from build123d import *

# Parameters (mm, degrees)
SKETCH1_W                = 38
SKETCH1_H                = 20
BOSS_EXTRUDE1_DEPTH      = 3
M3_CLEARANCE_HOLE1_D     = 3.2
M3_CLEARANCE_HOLE1_DEPTH = 20
M3_CLEARANCE_HOLE1_TIP   = 0.96137699
CUT_EXTRUDE1_DEPTH       = 3
FILLET1_R                = 1


with BuildPart() as part:
    # Sketch1 → Boss-Extrude1 (new body)
    with BuildSketch(Plane.XY):
        with Locations((-19, 10)):
            Rectangle(SKETCH1_W, SKETCH1_H)
    extrude(amount=BOSS_EXTRUDE1_DEPTH)

    # M3 Clearance Hole1
    with Locations(Plane.XY.offset(3)):
        with Locations((-11.25, 16), (-26.75, 16)):
            Hole(M3_CLEARANCE_HOLE1_D / 2, depth=M3_CLEARANCE_HOLE1_DEPTH)
            with Locations((0, 0, -(M3_CLEARANCE_HOLE1_DEPTH + M3_CLEARANCE_HOLE1_TIP / 2))):  # 118° drill point
                Cone(0, M3_CLEARANCE_HOLE1_D / 2, M3_CLEARANCE_HOLE1_TIP, mode=Mode.SUBTRACT)

    # Sketch4 → Cut-Extrude1 (cut)
    with BuildSketch(Plane.XY.offset(3)):
        with BuildLine():
            Line((-9.75, 5.03), (-28.25, 5.03))
            ThreePointArc((-28.25, 5.03), (-29.25, 4.03), (-28.25, 3.03))
            Line((-28.25, 3.03), (-9.75, 3.03))
            ThreePointArc((-9.75, 3.03), (-8.75, 4.03), (-9.75, 5.03))
        make_face()
    extrude(amount=-CUT_EXTRUDE1_DEPTH, mode=Mode.SUBTRACT)

    # Fillet1
    fillet1_edges = [part.edges().sort_by_distance(p)[0] for p in [
        (0, 0, 1.5),
        (-38, 0, 1.5),
        (-38, 20, 1.5),
        (0, 20, 1.5),
    ]]
    fillet(fillet1_edges, radius=FILLET1_R)


solid = part.part
Geometry: final body of the model. Coordinates: model frame, mm. A direction names the side the tool comes from. Round coordinates to 2 decimals unless told otherwise and drop trailing zeros. Loops run counter-clockwise (first coordinate to the right, second up) from the corner with the lowest first, then second, coordinate; pieces in that order, holes last.
Q1. Section D-D on y = 16. Return loops of the section in (x, z).
Q2. Section C-C on z = 1.2. Return loops of the section in (x, y).
Q3. Pull-direction query (X, two-part tool) for faces 3 (the cylindrical face through (-0.301, 0.285, 1.521)), 4 (the cylindrical face through (-37.715, 19.699, 1.521)), 5 (the flat face through (-19, 3.03, 2)); classes: released by +X, released by -X, zero draft, split by the parting line, or undercut.
Q4. Section A-A on x = -21. Return loops of the section in (y, z).
Q5. Section B-B on y = 4.03. Return loops of the section in (x, z).
Q6. Material intervals for L1, parallel to Y at x = -26.75, z = 1.8; L2, parallel to Y at x = -21, z = 0.3; L3, parallel to X at y = 4.75, z = 0.6, sorted ascending.
Q7. Access query for faces 1 (the flat face through (-19, 20, 1)), 2 (the cylindrical face through (-8.75, 4.01, 1.52)). Directions: +Z, -Z, +X, -X, +Y, -Y. A direction counts if a zero-diameter tool reaches every point of the face in a straight line with its end or side. Return the directions, or none.
Q8. Pin query (flat end, axial travel): P1, Ø12, axis at x = -21, y = 7, coming from the -Z side; P2, Ø3, axis at x = -11.25, y = 16, coming from the +Z side. Return the tip coordinate at first contact, or that it passes through.
Evaluation:
1. outline: (-38, 0) - (-28.35, 0) - (-28.35, 3) - (-38, 3) - close; (-25.15, 0) - (-12.85, 0) - (-12.85, 3) - (-25.15, 3) - close; (-9.65, 0) - (0, 0) - (0, 3) - (-9.65, 3) - close
2. outline: (-38, 1) arc R1 ccw to (-37, 0) - (-1, 0) arc R1 ccw to (0, 1) - (0, 19) arc R1 ccw to (-1, 20) - (-37, 20) arc R1 ccw to (-38, 19) - close; hole circle Ø3.2 at (-26.75, 16); hole (-28.25, 3.03) - (-9.75, 3.03) arc R1 ccw to (-9.75, 5.03) - (-28.25, 5.03) arc R1 ccw to start; hole circle Ø3.2 at (-11.25, 16)
3. face 3: released by +X
3. face 4: released by -X
3. face 5: undercut
4. outline: (0, 0) - (3.03, 0) - (3.03, 3) - (0, 3) - close; (5.03, 0) - (20, 0) - (20, 3) - (5.03, 3) - close
5. outline: (-38, 0) - (-29.25, 0) - (-29.25, 3) - (-38, 3) - close; (-8.75, 0) - (0, 0) - (0, 3) - (-8.75, 3) - close
6. L1: y = 0 to 3.03, 5.03 to 14.4, 17.6 to 20
6. L2: y = 0 to 3.03, 5.03 to 20
6. L3: x = -38 to -28.94, -9.06 to 0
7. face 1: +Z, -Z, +X, -X, +Y
7. face 2: +Z, -Z
8. P1: stops at z = 0
8. P2: passes through
